```python
from build123d import *

# Parameters (mm, degrees)
SKETCH3_W           = 86.5
SKETCH3_H           = 15
BOSS_EXTRUDE1_DEPTH = 13
SKETCH4_W           = 8.5
SKETCH4_H           = 12
CUT_EXTRUDE1_DEPTH  = 7
LPATTERN1_COUNT     = 9
LPATTERN1_PITCH     = 9.5
FILLET1_R           = 2
SKETCH5_R           = 2
CUT_EXTRUDE2_DEPTH  = 89.069574769
LPATTERN2_COUNT     = 9
LPATTERN2_PITCH     = 9.5


with BuildPart() as part:
    # Sketch3 → Boss-Extrude1 (new body)
    with BuildSketch(Plane(origin=(0, 0, 0), x_dir=(1, 0, 0), z_dir=(0, 1, 0))):
        with Locations((43.25, 7.5)):
            Rectangle(SKETCH3_W, SKETCH3_H)
    extrude(amount=BOSS_EXTRUDE1_DEPTH)

    # Sketch4 → Cut-Extrude1 (cut)
    with BuildSketch(Plane(origin=(0, 13, 0), x_dir=(1, 0, 0), z_dir=(0, 1, 0))):
        with Locations((5.25, 6)):
            Rectangle(SKETCH4_W, SKETCH4_H)
    cut_extrude1 = extrude(amount=-CUT_EXTRUDE1_DEPTH, mode=Mode.SUBTRACT)

    # LPattern1: Cut-Extrude1 ×9
    with Locations(*[(i * LPATTERN1_PITCH, 0, 0) for i in range(1, LPATTERN1_COUNT)]):
        add(cut_extrude1, mode=Mode.SUBTRACT)

    # Fillet1
    fillet1_edges = [part.edges().sort_by_distance(p)[0] for p in [
        (76.5, 13, 0),
        (86, 13, 0),
        (10, 13, 0),
        (19.5, 13, 0),
        (29, 13, 0),
        (38.5, 13, 0),
        (48, 13, 0),
        (0.5, 13, 0),
        (57.5, 13, 0),
        (67, 13, 0),
    ]]
    fillet(fillet1_edges, radius=FILLET1_R)

    # Sketch5 → Cut-Extrude2 (cut, through all)
    with BuildSketch(Plane(origin=(0, 6, 0), x_dir=(1, 0, 0), z_dir=(0, 1, 0))):
        with Locations(Location((5.25, 6, 0), (0, 0, 270))):
            Circle(SKETCH5_R)
    cut_extrude2 = extrude(amount=-CUT_EXTRUDE2_DEPTH, mode=Mode.SUBTRACT)

    # LPattern2: Cut-Extrude2 ×9
    with Locations(*[(i * LPATTERN2_PITCH, 0, 0) for i in range(1, LPATTERN2_COUNT)]):
        add(cut_extrude2, mode=Mode.SUBTRACT)


solid = part.part
```
CAD build for the part. Positions are in the model's coordinates, mm. A direction names the side the tool comes from. Coordinates: 2 decimals unless noted, no trailing zeros. Write each loop counter-clockwise with the first axis right and the second up, starting at its lowest first coordinate (ties: lowest second). Pieces come first, ordered by that corner, then holes. Notation, with made-up numbers: (86, 57.5) -> (102, 57.5) arc R34 cw to (102, 91.5) -> close; hole circle Ø11 at (66, 70). An arc over 180 degrees is marked (long way). Use CSV: the item, a comma, the result in double quotes. Start each with the question number.
Item 1: Band-saw the part on C-C, the plane x = 55.5. Write the cut outline in (y, z), plus the area to 3 significant figures.
Item 2: Wall check: probe 1 along Z at (x, y) = (33.5, 4.5); probe 2 along Y at (x, z) = (16.5, -9); probe 3 along Z at (x, y) = (69, 11.5). Give the ranges that are in metal, low to high.
Item 3: Two-plate mould, pull along X, no slides. Class faces 1 (the cylindrical face through (41.298, 3.042, -6.434)), 2 (the cylindrical face through (10.01, 12.4, -0.57)), 3 (the flat face through (0, 6, -7)): +X half, -X half, draft (parallel to the pull), parting line (faces both ways), or undercut.
Item 4: Band-saw the part on A-A, the plane x = 14.75. Write the cut outline in (y, z), plus the area to 3 significant figures.
Item 5: Tool access for faces 4 (the flat face through (15, 10, -12)), 5 (the flat face through (43, 6, -15)): list every direction of +Z, -Z, +X, -X, +Y, -Y with a clear straight run to the whole face (end or side of a thin tool).
Item 6: Band-saw the part on B-B, the plane y = 1.5. Give the number of separate pieces and of enclosed holes in the cut face, plus the area to 3 significant figures.
Item 7: Drop flat-ended pins along their axis: P1, Ø6.5, axis at x = 43.25, z = -6, coming from the +Y side; P2, Ø2.5, axis at x = 33.75, z = -6, coming from the -Y side; P3, Ø3.5, axis at x = 12.5, y = 11, coming from the +Z side. Give the stop position or say it passes through.
Response values:
1,outline,"(0, -15) -> (13, -15) -> (13, -12) -> (6, -12) -> (6, 0) -> (0, 0) -> close"
1,area,"111 mm2"
2,probe 1,"z = -15 to -7.98, -4.02 to 0"
2,probe 2,"y = 0 to 6"
2,probe 3,"z = -15 to -12"
3,face 1,"undercut"
3,face 2,"draft"
3,face 3,"-X half"
4,outline,"(0, -15) -> (13, -15) -> (13, -12) -> (6, -12) -> (6, -8) -> (0, -8) -> close; (0, -4) -> (6, -4) -> (6, 0) -> (0, 0) -> close"
4,area,"87.0 mm2"
5,face 4,"+Z, +Y"
5,face 5,"-Z, +X, -X, +Y, -Y"
6,separate pieces,"1"
6,enclosed holes,"9"
6,area,"1,180 mm2"
7,P1,"stops at y = 6"
7,P2,"passes through"
7,P3,"stops at z = -12"
